Check sheet for the drawn part. Datum: minimum x, y, z corner. Units: mm. A direction names the side the tool comes from. Coordinates: 2 decimals unless noted, no trailing zeros. Order: outer loops, then holes, each group sorted by start corner. A loop starts at its lowest first (then second) coordinate and runs counter-clockwise, first axis right, second up. Notation, with made-up numbers: (84, 60) - (137, 60) arc R26 ccw to (137, 82) - close; hole circle Ø5 at (13, 20.25). An arc over 180 degrees is marked (long way). Put each result on its own line as item: value.
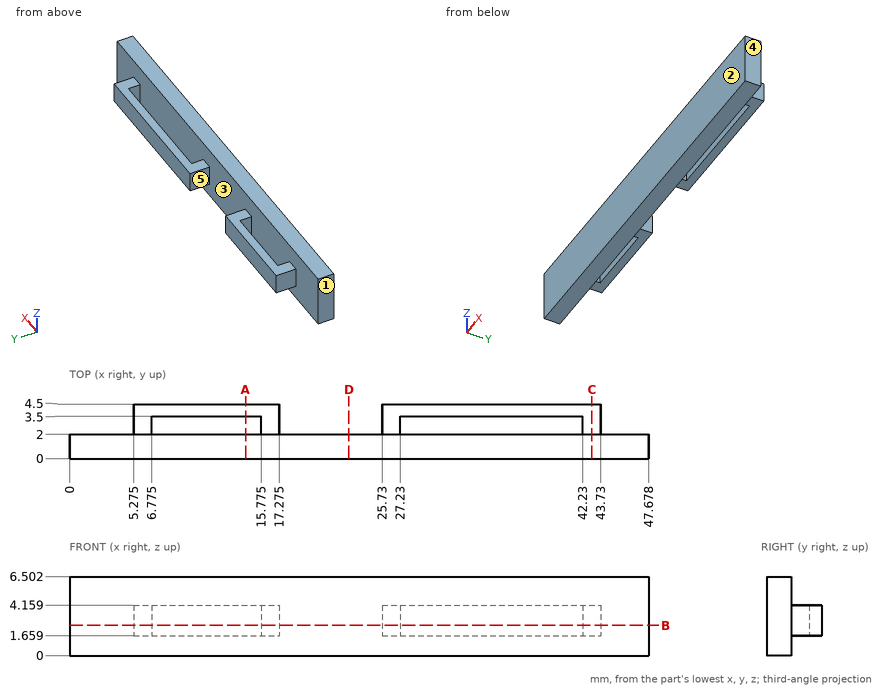
Q1. Section check D-D on x = 23. Record the boundary of the cut face in (y, z), then the cut area to 3 significant figures.
Answer block:
outline: (0, 0) - (2, 0) - (2, 6.5) - (0, 6.5) - close
area: 13.0 mm^2
Q2. Thickness scan on L1, parallel to X at y = 4, z = 2.75 (1 decimal); L2, parallel to Y at x = 34, z = 2; L3, parallel to Y at x = 17.5, z = 5.25. Record the ranges inside material, lowest first. Write a range as [from, to].
Answer block:
L1: x = [5.3, 17.3], [25.7, 43.7]
L2: y = [0, 2], [3.5, 4.5]
L3: y = [0, 2]
Q3. Depth check by flat-ended pin: pin 1 Ø1.2 at (x, z) = (33.5, 3) entering from -Y; pin 2 Ø1.2 at (y, z) = (3, 2.5) entering from +X; pin 3 Ø0.8 at (y, z) = (3.5, 2.5) entering from -X (1 decimal); pin 4 Ø1.2 at (x, y) = (12.5, 3) entering from +Z. Enter the tip coordinate at first touch or a pass-through.
Answer block:
pin 1: stops at y = 0
pin 2: stops at x = 43.73
pin 3: stops at x = 5.3
pin 4: stops at z = 4.16
Q4. Access from +Z, -Z, +X, -X, +Y, -Y to the whole of each face (thin tool, end or side, straight path). Record for the marked faces 4 and 5.
Answer block:
face 4: +Z, -Z, +X, +Y, -Y
face 5: +Z, -Z, +Y
Q5. Draft check along Y on the marked faces 1, 2 and 3. Enter one of: pulls with the +Y half, pulls with the -Y half, needs draft (parallel to the pull), parting line crosses it, or undercut.
Answer block:
face 1: needs draft
face 2: pulls with the -Y half
face 3: undercut
Q6. Section check A-A on x = 14.5. Record the boundary of the cut face in (y, z), then the cut area to 3 significant figures.
Answer block:
outline: (0, 0) - (2, 0) - (2, 6.5) - (0, 6.5) - close; (3.5, 1.66) - (4.5, 1.66) - (4.5, 4.16) - (3.5, 4.16) - close
area: 15.5 mm^2
Q7. Section check C-C on x = 43. Record the boundary of the cut face in (y, z).
Answer block:
outline: (0, 0) - (2, 0) - (2, 1.66) - (4.5, 1.66) - (4.5, 4.16) - (2, 4.16) - (2, 6.5) - (0, 6.5) - close
Q8. Section check B-B on z = 2.5. Record the boundary of the cut face in (x, y) (1 decimal).
Answer block:
outline: (0, 0) - (47.7, 0) - (47.7, 2) - (43.7, 2) - (43.7, 4.5) - (25.7, 4.5) - (25.7, 2) - (17.3, 2) - (17.3, 4.5) - (5.3, 4.5) - (5.3, 2) - (0, 2) - close; hole (6.8, 2) - (15.8, 2) - (15.8, 3.5) - (6.8, 3.5) - close; hole (27.2, 2) - (42.2, 2) - (42.2, 3.5) - (27.2, 3.5) - close
